Read the model definition and answer for the solid it produces. Units are mm, in the model's axes. A direction names the side the tool comes from. Coordinates: 2 decimals unless noted, no trailing zeros. Loops run counter-clockwise (first coordinate to the right, second up) from the corner with the lowest first, then second, coordinate; pieces in that order, holes last. Notation, with made-up numbers: (-0.5, 0) -> (57.5, 0) arc R19 cw to (57.5, 35) -> close; hole circle Ø2 at (18, 66). An arc over 180 degrees is marked (long way). Answer as a JSON object with one key per item and string values. Group by question number.
Q1. Determine the mould class of faces 4 (the flat face through (-39, -3, 7)), 5 (the flat face through (-60.299, -6, 7)), 6 (the flat face through (-4, -3, 7)) for opening direction X: released by +X, released by -X, zero draft, split by the parting line, or undercut.
Q2. Each of these flat-tipped pins is pushed along its axis until it touches: P1, Ø2, axis at y = -8.5, z = 4, coming from the +X side; P2, Ø2, axis at x = 6.5, z = 8, coming from the -Y side; P3, Ø1.5, axis at x = -44, z = 10, coming from the +Y side. Where does it stop, or does it pass through?
Q3. Straight lines are drawn through the part: line 1 along X through (y, z) = (-7.5, 1.25); line 2 along X through (y, z) = (-5, 12); line 3 along Y through (x, z) = (-31, 14.25). For each, find the intervals that lie inside material, in ascending order. Write a range as [from, to].
Q4. For faces 1 (the flat face through (6, -3, 7)), 2 (the flat face through (0, -2, 7)), 3 (the flat face through (-6.7, -1.5, 7.4)), determine the directions among +Z, -Z, +X, -X, +Y, -Y from which every point of the face is accessible in a straight line to the end or side of a thin tool.
Q5. The part is cut by section A-A on y = -7.25. Write down the section's boundary in (x, z), and give its area (3 significant figures).
Q6. The part is cut by section B-B on x = -40.5. Write down the section's boundary in (y, z), and give its area (3 significant figures).
Autodesk Inventor part; units mm, degrees
ref_plane "YZ Plane" through (0, 0, 0) normal (1, 0, 0) x (0, 1, 0)
ref_plane "XZ Plane" through (0, 0, 0) normal (0, 1, 0) x (-1, 0, 0)
ref_plane "XY Plane" through (0, 0, 0) normal (0, 0, 1) x (1, 0, 0)
sketch "Эскиз1" plane through (0, 0, 0) normal (0, 0, 1) x (1, 0, 0)
  line L0 (0, 0) -> (1, 0)
  line L1 (9, 0) -> (9, -3) construction
  line L2 (9, -3) -> (3.5, -3) construction
  line L3 (0, -3) -> (0, 0)
  line L4 (0, -3) -> (-7.3989, -3)
  line L5 (-7.3989, -3) -> (-7.3989, -6) construction
  line L6 (-7.3989, -6) -> (0, -6)
  line L7 (0, -6) -> (0, -3) construction
  line L8 (0, -3) -> (2.5, -3) construction
  line L9 (2.5, -4) -> (2.5, -5)
  line L10 (1.5, -6) -> (0, -6)
  line L11 (0, -6) -> (0, -3) construction
  line L12 (-7.3989, -3) -> (-6, 0)
  line L13 (-7.3989, -3) -> (-13.5, -3) construction
  line L14 (-57.3989, -3) -> (-57.3989, -6) construction
  line L15 (-57.3989, -6) -> (-7.3989, -6)
  line L16 (-7.3989, -6) -> (-7.3989, -3) construction
  arc A0 (1.5, -6) -> (2.5, -5) centre (1.5, -5) ccw
  arc A1 (3.5, -3) -> (2.5, -4) centre (3.5, -4) ccw
  line L17 (-13.5, -3) -> (-17.5, -3) construction
  line L18 (0, 0) -> (1, 0)
  line L19 (9, 0) -> (8, 0) construction
  arc A2 (1, 0) -> (8, 0) centre (4.5, 9.3675) ccw construction
  line L20 (-57.3989, -3) -> (-60.2989, -3)
  line L21 (-60.2989, -3) -> (-60.2989, -13)
  line L22 (-60.2989, -13) -> (-57.3989, -13) construction
  line L23 (-57.3989, -13) -> (-57.3989, -10) construction
  line L24 (-57.3989, -13) -> (8.6011, -13)
  line L25 (8.6011, -13) -> (8.6011, -10)
  line L26 (8.6011, -10) -> (-57.3989, -10)
  line L27 (-57.3989, -10) -> (-57.3989, -13) construction
  line L28 (-57.3989, -6) -> (-57.3989, -3) construction
  line L29 (-57.3989, -10) -> (-57.3989, -6)
  line L30 (-13.5, -3) -> (-17.5, -3) construction
  line L31 (-17.5, -3) -> (-57.3989, -3)
  line L32 (1, 0) -> (8, 0) construction
  line L33 (8, 0) -> (9, 0) construction
  line L34 (-57.3989, -13) -> (-60.2989, -13)
  line L35 (-60.2989, -13) -> (-60.2989, -13) construction
  line L36 (-6, 0) -> (-7.5, 0) construction
  line L37 (-7.5, 0) -> (-7.5, -3) construction
  line L38 (-7.5, 0) -> (-9.5, 0) construction
  line L39 (-7.5, 0) -> (-9.5, 0) construction
  line L40 (-9.5, 0) -> (-13.5, -3) construction
  line L41 (-13.5, -3) -> (-17.5, -3) construction
  spline S0 degree 3 poles (-7.5, 0) (-9.5, 0) (-13.5, -3) (-17.5, -3) knots 1 1 1 1 2 2 2 2
  line L42 (-7.5, 0) -> (-6, 0)
  line L43 (9, -3) -> (11, -3) construction
  line L44 (11, 0) -> (11, 1.5)
  line L45 (11, 1.5) -> (10.6727, 1.5)
  arc A3 (1, 0) -> (10.6727, 1.5) centre (4.5, 9.3675) ccw
  line L46 (3.5, -3) -> (8, -3)
  arc A4 (8, -3) -> (11, 0) centre (8, 0) ccw
  point P0 (2.5, -6)
  point P1 (0, -6)
  point P2 (2, -4)
  dimension "d0" = 9
  dimension "d1" = 3
  dimension "d3" = 3
  dimension "d4" = 2.5
  dimension "d5" = 3
  dimension "d6" = 50
  dimension "d9" = 1
  dimension "d10" = 1
  dimension "d11" = 4
  dimension "d13" = 3
  dimension "d14" = 1
  dimension "d15" = 1
  dimension "d16" = 10
  dimension "d17" = 2.9
  dimension "d18" = 10
  dimension "d20" = 3
  dimension "d21" = 66
  dimension "d25" = 4
  dimension "d26" = 66
  dimension "d27" = 90
  dimension "d28" = 90
  dimension "d29" = 65
  dimension "d30" = 6
  dimension "d31" = 3
  dimension "d32" = 1.5
  dimension "d33" = 6
  dimension "d34" = 2
  dimension "d37" = 2
  dimension "d38" = 4.5
  dimension "d39" = 3
  dimension "d40" = 2.9
extrude "Выдавливание1" add sketch "Эскиз1" along normal blind 15
sketch "Эскиз3" plane through (0, 0, 15) normal (0, 0, 1) x (1, 0, 0)
  line L0 (-57.3989, -6) -> (1.5, -6) construction
  arc A0 (1.5, -6) -> (2.5, -5) centre (1.5, -5) ccw construction
  arc A1 (3.5, -3) -> (2.5, -4) centre (3.5, -4) ccw construction
  line L1 (1, 0) -> (0, 0) construction
  line L2 (0, 0) -> (0, -3) construction
  line L3 (0, -3) -> (-7.3989, -3) construction
  line L4 (-7.3989, -3) -> (-6, 0) construction
  line L5 (-6, 0) -> (-7.5, 0) construction
  line L6 (-17.5, -3) -> (-60.2989, -3) construction
  line L7 (-60.2989, -3) -> (-60.2989, -13) construction
  line L8 (-60.2989, -13) -> (8.6011, -13) construction
  line L9 (8.6011, -13) -> (8.6011, -10) construction
  line L10 (8.6011, -10) -> (-57.3989, -10) construction
  line L11 (-57.3989, -10) -> (-57.3989, -6) construction
  line L12 (8.6011, -10) -> (-57.3989, -10) construction
  line L13 (-57.3989, -10) -> (-60.2989, -10)
  line L14 (-57.3989, -10) -> (11.5916, -5.7468)
  line L15 (11.5916, -5.7468) -> (11.9856, -17.8215)
  line L16 (11.9856, -17.8215) -> (-64.6581, -17.3068)
  line L17 (-64.6581, -17.3068) -> (-62.6934, -10.3264)
  line L18 (-62.6934, -10.3264) -> (-60.2989, -10)
  line L19 (2.5, -5) -> (2.5, -4)
  line L20 (3.5, -3) -> (8, -3)
  arc A2 (8, -3) -> (11, 0) centre (8, 0) ccw
  line L21 (11, 0) -> (11, 1.5)
  line L22 (11, 1.5) -> (10.6727, 1.5)
  arc A3 (1, 0) -> (10.6727, 1.5) centre (4.5, 9.3675) ccw
extrude "Выдавливание2" cut sketch "Эскиз3" against normal blind 25
sketch "Эскиз4" plane through (0, 0, 15) normal (0, 0, 1) x (1, 0, 0)
  line L0 (-60.2989, -10) -> (-57.3989, -10) construction
  line L1 (-57.3989, -10) -> (-57.3989, -6) construction
  line L2 (-57.3989, -6) -> (1.5, -6) construction
  arc A0 (1.5, -6) -> (2.5, -5) centre (1.5, -5) ccw construction
  line L3 (2.5, -5) -> (2.5, -4) construction
  arc A1 (3.5, -3) -> (2.5, -4) centre (3.5, -4) ccw construction
  line L4 (3.5, -3) -> (8, -3) construction
  arc A2 (8, -3) -> (11, 0) centre (8, 0) ccw construction
  line L5 (11, 0) -> (11, 1.5) construction
  line L6 (11, 1.5) -> (10.6727, 1.5) construction
  arc A3 (1, 0) -> (10.6727, 1.5) centre (4.5, 9.3675) ccw construction
  line L7 (1, 0) -> (0, 0) construction
  line L8 (0, 0) -> (0, -3) construction
  line L9 (0, -3) -> (-7.3989, -3) construction
  line L10 (-7.3989, -3) -> (-6, 0) construction
  line L11 (-6, 0) -> (-7.5, 0) construction
  line L12 (-17.5, -3) -> (-60.2989, -3) construction
  line L13 (-60.2989, -3) -> (-60.2989, -10) construction
  arc A4 (1, 0) -> (10.6727, 1.5) centre (4.5, 9.3675) ccw construction
  line L14 (1, 0) -> (9, -3) construction
  line L15 (9, -3) -> (10.6727, 1.5) construction
  spline S0 degree 2 poles (1, 0) (9, -3) (10.6727, 1.5) knots 1 1 1 2 2 2 construction
  line L16 (1, 0) -> (10.6727, 1.5) construction
  line L17 (11, 1.5) -> (10.6727, 1.5)
  line L18 (11, 1.5) -> (10, 1.5)
  line L19 (1, 0) -> (9, -3) construction
  line L20 (9, -3) -> (10, 1.5) construction
  spline S1 degree 2 poles (1, 0) (9, -3) (10, 1.5) knots 1 1 1 2 2 2
  line L21 (11, 0) -> (11, 1.5)
  line L22 (11, 1.5) -> (10, 0.696)
  line L23 (10, 0.696) -> (9.7197, 0.6526)
  line L24 (1, 0) -> (10, 1.5)
  dimension "d43" = 1
extrude "Выдавливание3" add sketch "Эскиз4" against normal up to surface (15 mm away) contours L22 L23 S1 L18 L17
extrude "Выдавливание4" cut sketch "Эскиз4" against normal up to surface (15 mm away) contours S1 L24
properties part number "bat_lock03_straight"
Final values:
{
 "1": {"face 4": "zero draft", "face 5": "released by -X", "face 6": "undercut"},
 "2": {"P1": "stops at x = -57.4", "P2": "stops at y = -3", "P3": "stops at y = -3"},
 "3": {"line 1": "x = [-60.3, -57.4]", "line 2": "x = [-60.3, 2.5]", "line 3": "y = [-6, -3]"},
 "4": {"face 1": "+Z, -Z, +X, -Y", "face 2": "+Z, -Z, +Y", "face 3": "+Z, -Z"},
 "5": {"outline": "(-60.3, 0) -> (-57.4, 0) -> (-57.4, 15) -> (-60.3, 15) -> close", "area": "43.5 mm2"},
 "6": {"outline": "(-6, 0) -> (-3, 0) -> (-3, 15) -> (-6, 15) -> close", "area": "45.0 mm2"}
}
